Build history of the part. All positions in model axes, mm. A direction names the side the tool comes from. Give positions to 0.01 mm unless a question says otherwise; leave off trailing zeros. Order: outer loops, then holes, each group sorted by start corner. A loop starts at its lowest first (then second) coordinate and runs counter-clockwise, first axis right, second up. Notation, with made-up numbers: (55.25, -34) - (108.25, -34) arc R25 ccw to (108.25, -9) - close; hole circle Ø2 at (59.5, 46). An arc over 180 degrees is marked (long way). Use a Markdown table: item, result.
from build123d import *

# Parameters (mm, degrees)
F0_R     = 2.375
F1_DEPTH = 10
F2_R     = 1.6
F3_DEPTH = 25.4
F4_SIZE  = 1.5
F5_SIZE  = 1


with BuildPart() as f1:
    # F0 (on Top) → F1 (new body)
    with BuildSketch(Plane.XY):
        with BuildLine():
            ThreePointArc((4.334937, 51), (0, 54.847421), (-4.334937, 51))
            Line((-4.334937, 51), (-4.334937, 44))
            Line((-4.334937, 44), (-6.457987, 42.022876))
            Line((-6.457987, 42.022876), (-6.457987, -52.157663))
            Line((-6.457987, -52.157663), (0, -52.157663))
            Line((0, -52.157663), (6.457987, -52.157663))
            Line((6.457987, -52.157663), (6.457987, 42.022876))
            Line((6.457987, 42.022876), (4.334937, 44))
            Line((4.334937, 44), (4.334937, 51))
        make_face()
        with Locations((0, -47.5)):
            Circle(F0_R, mode=Mode.SUBTRACT)
        with BuildLine():
            ThreePointArc((3.021839, 48.254199), (3.035714, 47.964286), (3.021839, 47.674372))
            Line((3.021839, 47.674372), (3.021839, 47.325628))
            ThreePointArc((3.021839, 47.325628), (3.035714, 47.035714), (3.021839, 46.745801))
            ThreePointArc((3.021839, 46.745801), (-0.06736, 44.000747), (-3.031726, 46.880157))
            ThreePointArc((-3.031726, 46.880157), (-3.035701, 47.044547), (-3.03077, 47.208911))
            Line((-3.03077, 47.208911), (-3.029152, 47.76479))
            ThreePointArc((-3.029152, 47.76479), (-0.244732, 50.990119), (3.021839, 48.254199))
        make_face(mode=Mode.SUBTRACT)
    extrude(amount=F1_DEPTH)

    # F2 (on Right) → F3 (cut)
    with BuildSketch(Plane.YZ):
        with Locations((47.519322, 5.252215)):
            Circle(F2_R)
    extrude(amount=F3_DEPTH, mode=Mode.SUBTRACT)

    # F4
    f4_edges = [f1.edges().sort_by_distance(p)[0] for p in [
        (6.457987, -5.067393, 10),
        (-6.457987, -5.067393, 10),
        (6.457987, -5.067393, 0),
        (-6.457987, -5.067393, 0),
    ]]
    chamfer(f4_edges, length=F4_SIZE)

    # F5
    f5_edges = [f1.edges().sort_by_distance(p)[0] for p in [
        (0, -52.157663, 0),
        (0, -52.157663, 10),
    ]]
    chamfer(f5_edges, length=F5_SIZE)


solid = f1.part
1) Slice it at B-B (y = -47.5). Write the cut outline in (x, z) (3 decimals).
Computed:
| item | result |
|---|---|
| outline | (-6.458, 1.5) - (-4.958, 0) - (-2.375, 0) - (-2.375, 10) - (-4.958, 10) - (-6.458, 8.5) - close; (2.375, 0) - (4.958, 0) - (6.458, 1.5) - (6.458, 8.5) - (4.958, 10) - (2.375, 10) - close |
2) Pin check, flat tips, straight feed: P1, Ø1.5, axis at x = -3.5, z = 4.5, coming from the +Y side; P2, Ø2, axis at y = 48.5, z = 5, coming from the -X side; P3, Ø4.5, axis at x = 0, y = -47.5, coming from the -Z side; P4, Ø2, axis at x = -3, z = 7, coming from the +Y side. Stop position of each tip, or through.
Computed:
| item | result |
|---|---|
| P1 | stops at y = 53.87 |
| P2 | stops at x = -4.33 |
| P3 | passes through |
| P4 | stops at y = 54.36 |
3) Two-plate mould, pull along Y, no slides. Class faces 1 (the cylindrical face through (-0.51, -49.82, 4.93)), 2 (the flat face through (5.41, 43, 4.93)), 3 (the flat face through (0, 3, 10)): +Y half, -Y half, draft (parallel to the pull), parting line (faces both ways), or undercut.
Computed:
| item | result |
|---|---|
| face 1 | undercut |
| face 2 | +Y half |
| face 3 | draft |
4) Slice it at A-A (x = 0). Write the cut outline in (y, z) (3 decimals), and give its area (3 significant figures).
Computed:
| item | result |
|---|---|
| outline | (-52.158, 1) - (-51.158, 0) - (-49.875, 0) - (-49.875, 10) - (-51.158, 10) - (-52.158, 9) - close; (-45.125, 0) - (44, 0) - (44, 10) - (-45.125, 10) - close; (51, 0) - (54.847, 0) - (54.847, 10) - (51, 10) - close |
| area | 952 mm² |
5) Slice it at C-C (y = 16). Write the cut outline in (x, z).
Computed:
| item | result |
|---|---|
| outline | (-6.46, 1.5) - (-4.96, 0) - (4.96, 0) - (6.46, 1.5) - (6.46, 8.5) - (4.96, 10) - (-4.96, 10) - (-6.46, 8.5) - close |
6) Tool access for faces 4 (the flat face through (-4.335, 48, 5)), 5 (the cylindrical face through (3.56, 49.045, 5.733)), 6 (the cylindrical face through (0, 44, 5)), 7 (the flat face through (4.335, 46, 4)), 8 (the flat face through (-6.458, -4, 5)): list every direction of +Z, -Z, +X, -X, +Y, -Y with a clear straight run to the whole face (end or side of a thin tool).
Computed:
| item | result |
|---|---|
| face 4 | +Z, -Z, -X, +Y |
| face 5 | +X |
| face 6 | +Z, -Z |
| face 7 | +Z, -Z, +X, +Y |
| face 8 | +Z, -Z, -X, +Y, -Y |
7) Wall check: line 1 (Y direction, x = 0, z = 6) (3 decimals); line 2 (X direction, y = 47.5, z = 7.75); line 3 (Y direction, x = -1, z = 9.5). Give the ranges that are in metal, low to high. Write a range as from..to.
Computed:
| item | result |
|---|---|
| line 1 | y = -52.158..-49.875, -45.125..44, 51..54.847 |
| line 2 | x = -4.33..-3.03, 3.02..4.33 |
| line 3 | y = -51.66..-49.65, -45.35..44.17, 50.83..54.73 |
